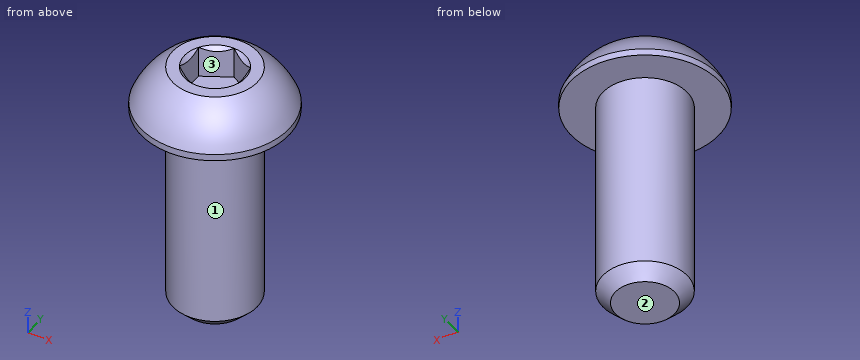
```python
from build123d import *

# Parameters (mm, degrees)
SKETCH1_W          = 15.875
SKETCH1_H          = 3.175
CHAMFER1_SIZE      = 0.9525
CUT_EXTRUDE2_DEPTH = 2.34696


with BuildPart() as part:
    # Sketch1 → Revolve1 (revolve)
    with BuildSketch(Plane(origin=(0, 0, 0), x_dir=(0, 0, -1), z_dir=(1, 0, 0))):
        with Locations((11.2903, 1.5875)):
            Rectangle(SKETCH1_W, SKETCH1_H)
    revolve(axis=Axis((0, 0, -19.2278), (0, 0, 1)))

    # Chamfer1
    chamfer1_edges = [part.edges().sort_by_distance(p)[0] for p in [
        (0, -3.175, -19.2278),
    ]]
    chamfer(chamfer1_edges, length=CHAMFER1_SIZE)

    # Sketch7 → Revolve2 (revolve)
    with BuildSketch(Plane(origin=(0, 0, 0), x_dir=(0, 0, -1), z_dir=(1, 0, 0)), mode=Mode.PRIVATE) as revolve2_sk:
        with BuildLine():
            Line((2.84988, 5.5499), (3.3528, 5.5499))
            Line((3.3528, 5.5499), (3.3528, 0))
            Line((3.3528, 0), (0, 0))
            Line((0, 0), (0, 3.175))
            ThreePointArc((0, 3.175), (1.235921075, 4.58927271), (2.84988, 5.5499))
        make_face()
    revolve(revolve2_sk.sketch.rotate(Axis((0, 0, 0), (0, 0, -1)), 180), axis=Axis((0, 0, 0), (0, 0, -1)))

    # Sketch5 → Cut-Extrude2 (cut)
    with BuildSketch(Plane.XY):
        Polygon((1.984375, -1.14567944), (1.984375, 1.14567944), (0, 2.291358881), (-1.984375, 1.14567944), (-1.984375, -1.14567944), (0, -2.291358881), align=None)
    extrude(amount=-CUT_EXTRUDE2_DEPTH, mode=Mode.SUBTRACT)

    # Cut-Extrude3 cone 1 section (on through the dimple's axis) → Cut-Extrude3 (revolve, cut)
    with BuildSketch(Plane(origin=(0, 0, 0), x_dir=(0, -1, 0), z_dir=(1, 0, 0))):
        Polygon((0, 0), (2.291358881, 0), (0, 2.291358881), align=None)
    revolve(axis=Axis((0, 0, 0), (0, 0, -1)), mode=Mode.SUBTRACT)


solid = part.part
```
Check sheet for the modelled part. Datum: model origin and axes. Units: mm. Face numbers are marked on the shaded views. Coordinates: 2 decimals unless noted, no trailing zeros. Order: outer loops, then holes, each group sorted by start corner. A loop starts at its lowest first (then second) coordinate and runs counter-clockwise, first axis right, second up. Notation, with made-up numbers: M 30,-31 L 76,-31 A27 ccw 76,-10 Z; hole C 20,52 d10. An arc over 180 degrees is marked long. Write each question's results on one line, items separated by ' | '. Start each with the question number.
1. Cross-section at D-D on x = 4.25. Record the cut outline in (y, z), and give its area (3 significant figures).
2. Cross-section at C-C on z = -13.75. Record the cut outline in (x, y) (3 decimals), and give its area (3 significant figures).
3. Cross-section at A-A on z = -2. Record the cut outline in (x, y).
4. Go/stop test with flat-tipped pins: P1, Ø1.8, axis at y = -0.5, z = -1, coming from the -X side; P2, Ø1, axis at x = 1, z = -16, coming from the -Y side; P3, Ø2, axis at x = 1, z = -11.5, coming from the +Y side (3 decimals); P4, Ø2.5, axis at y = 0, z = -2, coming from the +X side. Record where each tip stops, or that it passes through.
5. Cross-section at B-B on y = 0. Record the cut outline in (x, z) (1 decimal), and give its area (3 significant figures).
6. Material ranges on probe 1 along Y at (x, z) = (-0.5, -0.75); probe 2 along Z at (x, y) = (-0.25, -0.75); probe 3 along X at (y, z) = (1.5, -2), recorded low to high.
7. Mould release check, pull along Y, two halves, no side actions. Record for the marked faces 1, 2 and 3: +Y half, -Y half, draft (parallel to the pull), parting line (faces both ways), or undercut.
Checks:
1) outline: M -3.57,-3.35 L 3.57,-3.35 L 3.57,-2.85 A4.2 ccw -3.57,-2.85 Z | area: 13.6 mm²
2) outline: C 0,0 d6.35 | area: 31.7 mm²
3) outline: C 0,0 d10.26; hole M -1.98,-1.15 L 0,-2.29 L 1.98,-1.15 L 1.98,1.15 L 0,2.29 L -1.98,1.15 Z
4) P1: stops at x = -5.05 | P2: stops at y = -3.14 | P3: stops at y = 3.175 | P4: stops at x = 5.55
5) outline: M -5.5,-3.4 L -3.2,-3.4 L -3.2,-18.3 L -2.2,-19.2 L 2.2,-19.2 L 3.2,-18.3 L 3.2,-3.4 L 5.5,-3.4 L 5.5,-2.8 A6 ccw 3.2,0 L 2.3,0 L 2,-0.3 L 2,-2.3 L -2,-2.3 L -2,-0.3 L -2.3,0 L -3.2,0 A6 ccw -5.5,-2.8 Z | area: 122 mm²
6) probe 1: y = -4.11 to -2, 2 to 4.11 | probe 2: z = -19.23 to -2.35 | probe 3: x = -4.91 to -1.37, 1.37 to 4.91
7) face 1: parting line | face 2: draft | face 3: undercut
